Part model, mm, in its own coordinate system. A direction names the side the tool comes from. Coordinates: 2 decimals unless noted, no trailing zeros. Write each loop counter-clockwise with the first axis right and the second up, starting at its lowest first coordinate (ties: lowest second). Pieces come first, ordered by that corner, then holes. Notation, with made-up numbers: (6.5, 53.5) -> (21.5, 53.5) arc R5 cw to (21.5, 61.5) -> close; hole circle Ø5 at (-32.75, 2.5). An arc over 180 degrees is marked (long way). Write item = value, one per line.
from build123d import *

# Parameters (mm, degrees)
SKETCH1_W           = 80
SKETCH1_H           = 40
SKETCH1_W_2         = 76
SKETCH1_H_2         = 36
BOSS_EXTRUDE1_DEPTH = 100
SKETCH2_R           = 4
SKETCH2_R_2         = 5
CUT_EXTRUDE1_DEPTH  = 40
SKETCH3_R           = 3
CUT_EXTRUDE2_DEPTH  = 80


with BuildPart() as part:
    # Sketch1 → Boss-Extrude1 (new body)
    with BuildSketch(Plane(origin=(0, 0, 0), x_dir=(1, 0, 0), z_dir=(0, 1, 0))):
        with Locations((40, 20)):
            Rectangle(SKETCH1_W, SKETCH1_H)
        with Locations((40, 20)):
            Rectangle(SKETCH1_W_2, SKETCH1_H_2, mode=Mode.SUBTRACT)
    extrude(amount=BOSS_EXTRUDE1_DEPTH)

    # Sketch2 → Cut-Extrude1 (cut)
    with BuildSketch(Plane.XY):
        with Locations((70, 15)):
            Circle(SKETCH2_R)
        with Locations((70, 85)):
            Circle(SKETCH2_R)
        with Locations((10, 15)):
            Circle(SKETCH2_R)
        with Locations((10, 50)):
            Circle(SKETCH2_R_2)
        with Locations((10, 85)):
            Circle(SKETCH2_R)
        with Locations((70, 50)):
            Circle(SKETCH2_R_2)
    extrude(amount=-CUT_EXTRUDE1_DEPTH, mode=Mode.SUBTRACT)

    # Sketch3 → Cut-Extrude2 (cut)
    with BuildSketch(Plane.ZY):
        with Locations((-20, 30)):
            Circle(SKETCH3_R)
        with Locations((-20, 70)):
            Circle(SKETCH3_R)
    extrude(amount=-CUT_EXTRUDE2_DEPTH, mode=Mode.SUBTRACT)


solid = part.part
Q1. Probe line 1 (Y direction, x = 79.15, z = -20); line 2 (Z direction, x = 75, y = 32.5); line 3 (Y direction, x = 70, z = -1). List the from-to ranges inside material, lowest first. Write a range as from..to.
Model answer:
line_1 = 0..27, 33..67, 73..100
line_2 = -40..-38, -2..0
line_3 = 0..11, 19..45, 55..81, 89..100
Q2. Which spindle directions (+Z, -Z, +X, -X, +Y, -Y) get a long thin tool onto all of the face, cutting with end or side? Do faces 1 (the face through (78, 49, -20)), 2 (the face through (0, 49, -20)). Say none if no direction does.
Model answer:
face_1 = +Y, -Y
face_2 = +Z, -Z, -X, +Y, -Y
Q3. Mould opens along X. For faces 3 (the face through (9.133, 81.095, -0.986)), 4 (the face through (80, 49, -20)), 5 (the face through (39, 49, 0)) say: released by +X, released by -X, zero draft, split by the parting line, or undercut.
Model answer:
face_3 = undercut
face_4 = released by +X
face_5 = zero draft
Q4. Saw through at A-A on x = 10. Count the separate pieces of the cut face and the enclosed holes in it, and give its area (3 significant figures).
Model answer:
separate_pieces = 8
enclosed_holes = 0
area = 296 mm²
Q5. Saw through at D-D on z = -28.5. Give the cut face in (x, y), and give its area (3 significant figures).
Model answer:
outline = (0, 0) -> (2, 0) -> (2, 100) -> (0, 100) -> close; (78, 0) -> (80, 0) -> (80, 100) -> (78, 100) -> close
area = 400 mm²
Q6. Saw through at C-C on y = 22.5. Give the cut face in (x, z).
Model answer:
outline = (0, -40) -> (80, -40) -> (80, 0) -> (0, 0) -> close; hole (2, -38) -> (78, -38) -> (78, -2) -> (2, -2) -> close
Q7. Saw through at B-B on y = 50. Give the cut face in (x, z).
Model answer:
outline = (0, -40) -> (5, -40) -> (5, -38) -> (2, -38) -> (2, -2) -> (5, -2) -> (5, 0) -> (0, 0) -> close; (15, -40) -> (65, -40) -> (65, -38) -> (15, -38) -> close; (15, -2) -> (65, -2) -> (65, 0) -> (15, 0) -> close; (75, -40) -> (80, -40) -> (80, 0) -> (75, 0) -> (75, -2) -> (78, -2) -> (78, -38) -> (75, -38) -> close
